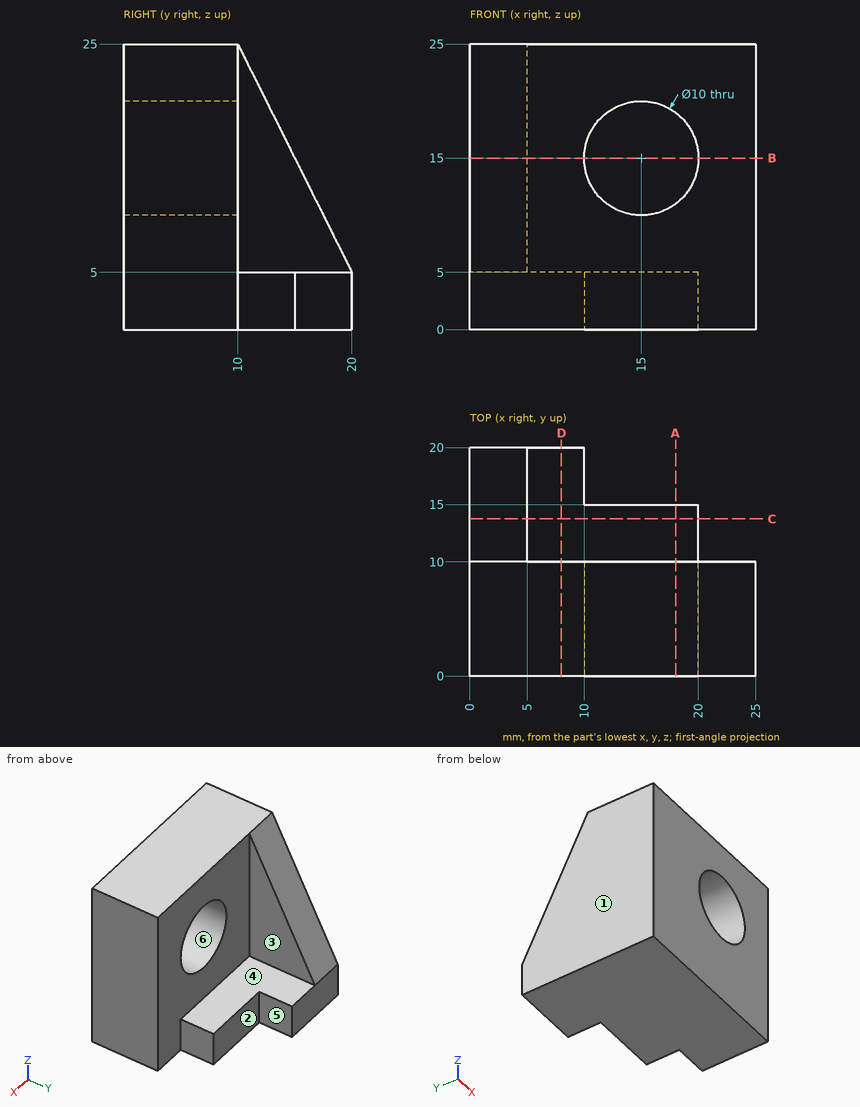
Print and shaded views of the part. All mm, measured from the part's lowest x, y and z. A direction names the side the tool comes from. Give positions to 0.01 mm unless a question says otherwise; leave off trailing zeros. Loops run counter-clockwise (first coordinate to the right, second up) from the corner with the lowest first, then second, coordinate; pieces in that order, holes last.
1) Saw through at B-B (z = 15). Write the cut outline in (x, y), plus the area to 3 significant figures.
2) Saw through at C-C (y = 13.75). Write the cut outline in (x, z), plus the area to 4 significant figures.
3) Wall check: line 1 (X direction, y = 2.5, z = 15); line 2 (Z direction, x = 9, y = 16.25). Give the ranges that are in metal, low to high.
4) Saw through at A-A (x = 18). Write the cut outline in (y, z), plus the area to 3 significant figures.
5) Flat gauge pins, fed straight in: pin 1 Ø1.5 at (y, z) = (18, 2) entering from +X; pin 2 Ø1.5 at (x, z) = (22.5, 20) entering from +Y; pin 3 Ø1.5 at (x, z) = (13.5, 2.5) entering from +Y. Where does each tip first touch, or does it go through?
6) Tool access for the marked faces 1, 2 and 3: list every direction of +Z, -Z, +X, -X, +Y, -Y with a clear straight run to the whole face (end or side of a thin tool).
7) Pull direction X, two halves, no side cores. Call the marked faces 4, 5 and 6: +X half, -X half, draft (parallel to the pull), parting line (faces both ways), or undercut.
8) Saw through at D-D (x = 8). Write the cut outline in (y, z).
Answer block:
1. outline: (0, 0) - (10, 0) - (10, 10) - (5, 10) - (5, 15) - (0, 15) - close; (20, 0) - (25, 0) - (25, 10) - (20, 10) - close
1. area: 175 mm2
2. outline: (0, 0) - (20, 0) - (20, 5) - (5, 5) - (5, 17.5) - (0, 17.5) - close
2. area: 162.5 mm2
3. line 1: x = 0 to 10, 20 to 25
3. line 2: z = 0 to 5
4. outline: (0, 0) - (15, 0) - (15, 5) - (10, 5) - (10, 11) - (0, 11) - close; (0, 19) - (10, 19) - (10, 25) - (0, 25) - close
4. area: 195 mm2
5. pin 1: stops at x = 10
5. pin 2: stops at y = 10
5. pin 3: stops at y = 15
6. face 1: +Z, -Z, -X, +Y, -Y
6. face 2: +Z, -Z, +X, +Y
6. face 3: +Z, +X, +Y
7. face 4: draft
7. face 5: +X half
7. face 6: undercut
8. outline: (0, 0) - (20, 0) - (20, 5) - (10, 5) - (10, 25) - (0, 25) - close
